Geometry check sheet. Reference: drawing and pictorial views, mm from the part's lowest x, y, z. A direction names the side the tool comes from. Give positions to 0.01 mm unless a question says otherwise; leave off trailing zeros. Loops run counter-clockwise (first coordinate to the right, second up) from the corner with the lowest first, then second, coordinate; pieces in that order, holes last. Notation, with made-up numbers: (21.5, 78.25) -> (77.5, 78.25) arc R18 ccw to (77.5, 95.25) -> close; hole circle Ø8 at (53.25, -0.75). An arc over 180 degrees is marked (long way). Answer in a Markdown table with one row per item. Add a question column.
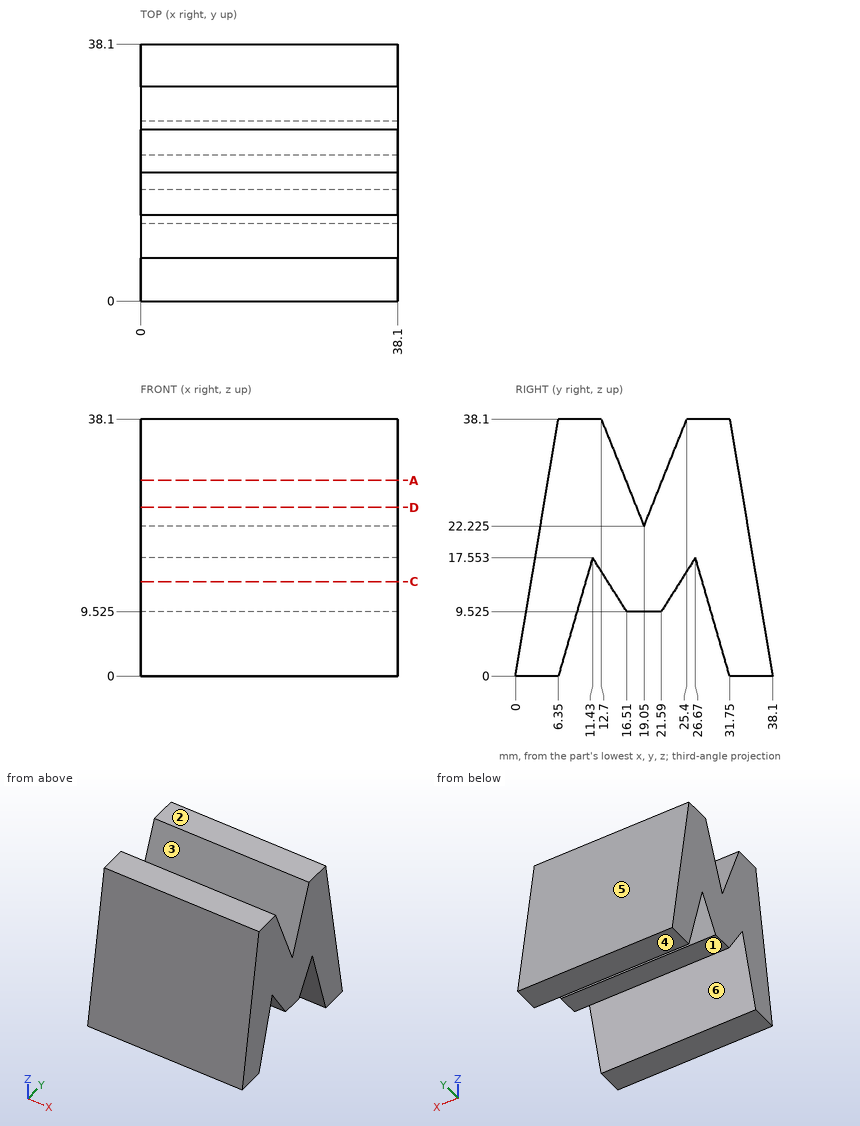
1. Material ranges on L1, parallel to Y at x = 33, z = 31.5; L2, parallel to Y at x = 21.5, z = 6; L3, parallel to Y at x = 31.5, z = 18, recorded low to high. Write a range as from..to.
2. Sectioned sample at D-D (z = 25). Enter the section's corners in (x, y), plus the area to 3 significant figures.
3. Sectioned sample at A-A (z = 29). Enter the section's corners in (x, y).
4. Sectioned sample at C-C (z = 14). Enter the section's corners in (x, y), plus the area to 3 significant figures.
5. Access from +Z, -Z, +X, -X, +Y, -Y to the whole of each face (thin tool, end or side, straight path). Record for the marked faces 1, 2 and 3.
6. Gauge pin test, flat ends, axial feed: pin 1 Ø2 at (x, z) = (13, 34) entering from -Y; pin 2 Ø2.5 at (x, y) = (27, 18) entering from -Z (3 decimals); pin 3 Ø12 at (x, z) = (11, 12) entering from -Y. Record the tip position at first contact, or that the pin passes through.
7. Release check for a two-part mould opening along Y. For the marked faces 4, 5 and 6 record: released by +Y, released by -Y, zero draft, split by the parting line, or undercut.
Response:
| question | item | result |
|---|---|---|
| 1 | L1 | y = 5.25..15.34, 22.76..32.85 |
| 1 | L2 | y = 1..8.09, 30.01..37.1 |
| 1 | L3 | y = 3..35.1 |
| 2 | outline | (0, 4.17) -> (38.1, 4.17) -> (38.1, 17.94) -> (0, 17.94) -> close; (0, 20.16) -> (38.1, 20.16) -> (38.1, 33.93) -> (0, 33.93) -> close |
| 2 | area | 1,050 mm2 |
| 3 | outline | (0, 4.83) -> (38.1, 4.83) -> (38.1, 16.34) -> (0, 16.34) -> close; (0, 21.76) -> (38.1, 21.76) -> (38.1, 33.27) -> (0, 33.27) -> close |
| 4 | outline | (0, 2.33) -> (38.1, 2.33) -> (38.1, 10.4) -> (0, 10.4) -> close; (0, 13.68) -> (38.1, 13.68) -> (38.1, 24.42) -> (0, 24.42) -> close; (0, 27.7) -> (38.1, 27.7) -> (38.1, 35.77) -> (0, 35.77) -> close |
| 4 | area | 1,020 mm2 |
| 5 | face 1 | -Z, +X, -X |
| 5 | face 2 | +Z, +X, -X, +Y, -Y |
| 5 | face 3 | +Z, +X, -X |
| 6 | pin 1 | stops at y = 5.5 |
| 6 | pin 2 | stops at z = 9.525 |
| 6 | pin 3 | stops at y = 1 |
| 7 | face 4 | zero draft |
| 7 | face 5 | released by +Y |
| 7 | face 6 | undercut |
